Read the model definition and answer for the solid it produces. Units are mm, in the model's axes. Face numbers are marked on the shaded views. A direction names the side the tool comes from. Give positions to 0.01 mm unless a question says otherwise; leave off trailing zeros. Write each loop counter-clockwise with the first axis right and the second up, starting at its lowest first coordinate (ties: lowest second). Pieces come first, ordered by that corner, then holes. Notation, with made-up numbers: (-30, 89) -> (24, 89) arc R5 ccw to (24, 97) -> close; hole circle Ø6 at (22, 78). An arc over 180 degrees is marked (long way). Write item = value, one per line.
from build123d import *

# Parameters (mm, degrees)
SKETCH1_R           = 39.6875
BOSS_EXTRUDE1_DEPTH = 12.7
FILLET1_R           = 12.7
FILLET2_R           = 3.175
SKETCH2_R           = 2.25
CUT_EXTRUDE1_DEPTH  = 69.538830235
CUT_EXTRUDE2_DEPTH  = 7.62
SKETCH9_R           = 2.25
CUT_EXTRUDE3_DEPTH  = 69.538830235


with BuildPart() as part:
    # Sketch1 → Boss-Extrude1 (new body)
    with BuildSketch(Plane(origin=(0, 0, 0), x_dir=(1, 0, 0), z_dir=(0, 1, 0))):
        with BuildLine():
            Line((-47.625, 0), (-47.625, 3.175))
            Line((-47.625, 3.175), (-41.275, 3.175))
            Line((-41.275, 3.175), (-41.275, 47.625))
            Line((-41.275, 47.625), (41.275, 47.625))
            Line((41.275, 47.625), (41.275, 3.175))
            Line((41.275, 3.175), (47.625, 3.175))
            Line((47.625, 3.175), (47.625, 0))
            ThreePointArc((47.625, 0), (0, -47.625), (-47.625, 0))
        make_face()
        with Locations(Location((0, 0, 0), (0, 0, 270))):
            Circle(SKETCH1_R, mode=Mode.SUBTRACT)
    extrude(amount=BOSS_EXTRUDE1_DEPTH)

    # Fillet1
    fillet1_edges = [part.edges().sort_by_distance(p)[0] for p in [
        (-41.275, 6.35, -47.625),
        (41.275, 6.35, -47.625),
    ]]
    fillet(fillet1_edges, radius=FILLET1_R)

    # Fillet2
    fillet2_edges = [part.edges().sort_by_distance(p)[0] for p in [
        (47.625, 6.35, -3.175),
        (-47.625, 6.35, -3.175),
    ]]
    fillet(fillet2_edges, radius=FILLET2_R - 0.0001)  # a hair under: the kernel refuses the full size

    # Sketch2 → Cut-Extrude1 (cut, through all)
    with BuildSketch(Plane(origin=(0, 12.7, 0), x_dir=(1, 0, 0), z_dir=(0, 1, 0))):
        with Locations(Location((-34.925, 34.925, 0), (0, 0, 270))):
            Circle(SKETCH2_R)
        with Locations(Location((34.925, 34.925, 0), (0, 0, 270))):
            Circle(SKETCH2_R)
    extrude(amount=-CUT_EXTRUDE1_DEPTH, mode=Mode.SUBTRACT)

    # Sketch6 → Cut-Extrude2 (cut)
    with BuildSketch(Plane(origin=(0, 12.7, 0), x_dir=(1, 0, 0), z_dir=(0, 1, 0))):
        with BuildLine():
            Line((-49.187681697, -31.694494567), (-48.884558606, -41.276047168))
            ThreePointArc((-48.884558606, -41.276047168), (-5.562483374, -46.004938144), (36.043462017, -33.039217165))
            ThreePointArc((36.043462017, -33.039217165), (48.826767021, 2.582217505), (32.357577485, 36.656625654))
            Line((32.357577485, 36.656625654), (-25.491069939, 87.720848233))
            ThreePointArc((-25.491069939, 87.720848233), (-29.666518146, 56.664530057), (-15.884572215, 28.522262332))
            ThreePointArc((-15.884572215, 28.522262332), (-10.696498958, -13.664606553), (-49.187681697, -31.694494567))
        make_face()
    extrude(amount=-CUT_EXTRUDE2_DEPTH, mode=Mode.SUBTRACT)

    # Sketch9 → Cut-Extrude3 (cut, through all)
    with BuildSketch(Plane(origin=(0, 12.7, 0), x_dir=(1, 0, 0), z_dir=(0, 1, 0))):
        with Locations(Location((-37.944903067, -21.9075, 0), (0, 0, 270))):
            Circle(SKETCH9_R)
    extrude(amount=-CUT_EXTRUDE3_DEPTH, mode=Mode.SUBTRACT)


solid = part.part
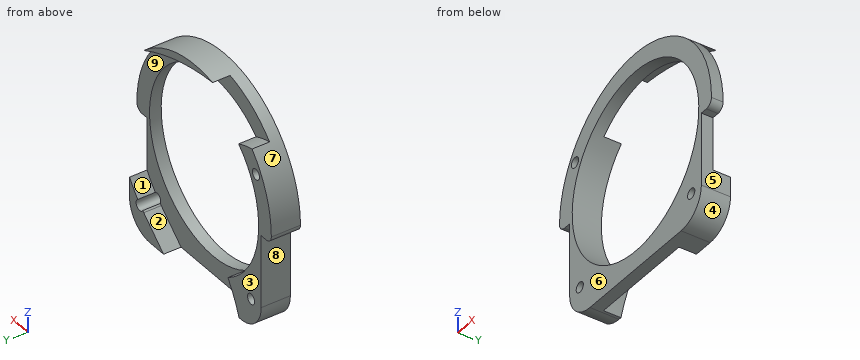
(1) The part is cut by section A-A on y = 8.5. Count the separate pieces of the cut face and the enclosed holes in it, plus the area to 3 significant figures.
Checks:
separate_pieces = 3
enclosed_holes = 2
area = 956 mm²
(2) For a pull along X with two mould halves and no side action, classify the marked faces 1, 2, 3 and 4 as released by +X, released by -X, zero draft, split by the parting line, or undercut.
Checks:
face_1 = undercut
face_2 = undercut
face_3 = zero draft
face_4 = released by +X
(3) Consider L1, parallel to X at y = 2.5, z = -35; L2, parallel to X at y = 1.75, z = 20.5; L3, parallel to X at y = 3, z = -31 (3 decimals). Determine where each line is inside the solid, lowest interval first.
Checks:
L1 = -41.27 to -37.17, -32.68 to -18.71, 18.71 to 32.68, 37.17 to 41.27
L2 = -42.99 to -39.7, -36.19 to -33.98, 33.98 to 42.99
L3 = -41.275 to -24.781, 24.781 to 41.275
(4) The part is cut by section D-D on z = -15.5. Determine the outline of the cut face in (x, y) (3 decimals).
Checks:
outline = (-41.275, 0) -> (-36.536, 0) -> (-36.536, 12.7) -> (-41.275, 12.7) -> close; (36.536, 0) -> (41.275, 0) -> (41.275, 5.08) -> (36.536, 5.08) -> close
(5) A tool of negligible diameter and unlimited length cuts with its end or side. For the marked faces 5, 6, 7, 8 and 9, from which of +Z, -Z, +X, -X, +Y, -Y can it reach the whole face along a straight path? Write none if from no direction.
Checks:
face_5 = -Z, +X, +Y, -Y
face_6 = +Z, -Z, +X, -X, -Y
face_7 = +Z, +Y, -Y
face_8 = -Z, -X, +Y, -Y
face_9 = +Y
(6) Given P1, Ø3, axis at x = 33, y = 3, coming from the +Z side; P2, Ø6.5, axis at y = 9, z = -11.5, coming from the +X side; P3, Ø4, axis at y = 4, z = -0.5, coming from the +X side (3 decimals); P4, Ø3, axis at x = -29, y = 2, coming from the +Z side, each flat-ended and moving along its own axis, determine where each tip first touches the part or whether it passes through.
Checks:
P1 = 35.72
P2 = -36.84
P3 = 47.625
P4 = 38.88
(7) The part is cut by section B-B on x = -18.5. Determine the outline of the cut face in (y, z) (3 decimals), plus the area to 3 significant figures.
Checks:
outline = (0, -47.625) -> (5.08, -47.625) -> (5.08, -35.112) -> (0, -35.112) -> close; (0, 35.112) -> (5.08, 35.112) -> (5.08, 43.885) -> (0, 43.885) -> close
area = 108 mm²
